For this review, take the finished solid that the model builds, in its own axes (mm). A direction names the side the tool comes from. Round coordinates to 2 decimals unless told otherwise and drop trailing zeros. Order: outer loops, then holes, each group sorted by start corner. A loop starts at its lowest first (then second) coordinate and runs counter-clockwise, first axis right, second up. Notation, with made-up numbers: M 81,65 L 123,65 A17 cw 123,95 Z; hole C 37.5,-8 d2. An arc over 180 degrees is marked long. Answer as a JSON object with one key per item and string values.
from build123d import *

# Parameters (mm, degrees)
BOSS_EXTRUDE1_DEPTH = 327.500000024


with BuildPart() as part:
    # Sketch1 → Boss-Extrude1 (new body)
    with BuildSketch(Plane.XY):
        Polygon((-22.499997904, -22.500007621), (-4.099997904, -22.500007621), (-4.099997904, -18.000007621), (-6.799997904, -18.000007621), (-6.799997904, -9.500007621), (-4.499997904, -7.200007621), (4.500002096, -7.200007621), (6.800002096, -9.500007621), (6.800002096, -18.000007621), (4.100002096, -18.000007621), (4.100002096, -22.500007621), (22.500002096, -22.500007621), (22.500002096, -4.100007621), (18.000002096, -4.100007621), (18.000002096, -6.800007621), (9.500002096, -6.800007621), (7.200002096, -4.500007621), (7.200002096, 4.499992379), (9.500002096, 6.799992379), (18.000002096, 6.799992379), (18.000002096, 4.099992379), (22.500002096, 4.099992379), (22.500002096, 22.499992379), (4.100002096, 22.499992379), (4.100002096, 17.999992379), (6.800002096, 17.999992379), (6.800002096, 9.499992379), (4.500002096, 7.199992379), (-4.499997904, 7.199992379), (-6.799997904, 9.499992379), (-6.799997904, 17.999992379), (-4.099997904, 17.999992379), (-4.099997904, 22.499992379), (-22.499997904, 22.499992379), (-22.499997904, 4.099992379), (-17.999997904, 4.099992379), (-17.999997904, 6.799992379), (-9.499997904, 6.799992379), (-7.199997904, 4.499992379), (-7.199997904, -4.500007621), (-9.499997904, -6.800007621), (-17.999997904, -6.800007621), (-17.999997904, -4.100007621), (-22.499997904, -4.100007621), align=None)
        Polygon((8.200003223, 8.199980186), (8.199989777, 19.399992368), (6.500002085, 19.399992368), (6.500002085, 21.099984758), (21.100004192, 21.099984758), (21.100004192, 6.499980188), (19.400009891, 6.499980188), (19.400009891, 8.199980186), align=None, mode=Mode.SUBTRACT)
        Polygon((-19.399997893, 6.499992368), (-21.099990283, 6.499992368), (-21.099990283, 21.099994475), (-6.499974376, 21.099994475), (-6.49997587, 19.399985233), (-8.199975868, 19.399986727), (-8.199985712, 8.19998006), (-19.399997893, 8.19998006), align=None, mode=Mode.SUBTRACT)
        Polygon((-6.499997893, -21.1), (-21.1, -21.1), (-21.1, -6.499995431), (-19.400002096, -6.499995431), (-19.400002096, -8.199995429), (-8.199995429, -8.199995429), (-8.199995429, -19.40000761), (-6.499997893, -19.400009104), align=None, mode=Mode.SUBTRACT)
        Polygon((6.499989905, -19.400011813), (8.199989903, -19.400011813), (8.199989903, -8.200005146), (19.400002085, -8.200005146), (19.400003579, -6.500017454), (21.099994475, -6.500018948), (21.099994475, -21.100009717), (6.499989905, -21.100009717), align=None, mode=Mode.SUBTRACT)
        with BuildLine():
            Line((-5.799999723, 3.537265469), (-3.451121085, 1.18838683))
            ThreePointArc((-3.451121085, 1.18838683), (-2.580942431, 2.580937072), (-1.188393996, 3.451118617))
            Line((-1.188393996, 3.451118617), (-3.537277512, 5.799992379))
            Line((-3.537277512, 5.799992379), (3.537277512, 5.799992379))
            Line((3.537277512, 5.799992379), (1.188393996, 3.451118617))
            ThreePointArc((1.188393996, 3.451118617), (2.580942431, 2.580937072), (3.451121085, 1.18838683))
            Line((3.451121085, 1.18838683), (5.799999723, 3.537265469))
            Line((5.799999723, 3.537265469), (5.799985034, -3.537266022))
            Line((5.799985034, -3.537266022), (3.451117181, -1.188398168))
            ThreePointArc((3.451117181, -1.188398168), (2.580938191, -2.580941312), (1.188393996, -3.451118617))
            Line((1.188393996, -3.451118617), (3.537277512, -5.799992379))
            Line((3.537277512, -5.799992379), (-3.537277512, -5.799992379))
            Line((-3.537277512, -5.799992379), (-1.188393996, -3.451118617))
            ThreePointArc((-1.188393996, -3.451118617), (-2.580938191, -2.580941311), (-3.451117181, -1.188398168))
            Line((-3.451117181, -1.188398168), (-5.799985034, -3.537266022))
            Line((-5.799985034, -3.537266022), (-5.799999723, 3.537265469))
        make_face(mode=Mode.SUBTRACT)
    extrude(amount=BOSS_EXTRUDE1_DEPTH)


solid = part.part
1) Insertion check: P1, Ø3, axis at y = 1, z = 275.5, coming from the +X side; P2, Ø3.5, axis at y = -1, z = 179.5, coming from the -X side. Each pin has a flat end and moves straight along its axis. Give the tip position at first contact, or say it passes through.
Geometry check:
{"P1": "stops at x = 7.2", "P2": "stops at x = -7.2"}
2) Machinability: for faces 1 (the flat face through (14, -6.8, 161)), 2 (the flat face through (22.5, 13, 161)), which of the approach directions +Z, -Z, +X, -X, +Y, -Y give a long, thin tool a straight path to every point of the face, cutting with its end or side? Answer none if there is none.
Geometry check:
{"face 1": "+Z, -Z", "face 2": "+Z, -Z, +X, +Y, -Y"}
3) Add section A-A on y = -14.5. State the section outline as (x, z) points, and give its area (3 significant figures).
Geometry check:
{"outline": "M -22.5,0 L -21.1,0 L -21.1,327.5 L -22.5,327.5 Z; M -8.2,0 L -6.8,0 L -6.8,327.5 L -8.2,327.5 Z; M 6.8,0 L 8.2,0 L 8.2,327.5 L 6.8,327.5 Z; M 21.1,0 L 22.5,0 L 22.5,327.5 L 21.1,327.5 Z", "area": "1,830 mm²"}
4) Mouldability with a two-part tool opening along Y and no side actions: class faces 3 (the flat face through (-14, -21.1, 161)), 4 (the flat face through (-13, -22.5, 161)), 5 (the flat face through (-3.4, 1.8, 327.5)) as +Y half, -Y half, draft (parallel to the pull), parting line (faces both ways), or undercut.
Geometry check:
{"face 3": "undercut", "face 4": "-Y half", "face 5": "draft"}
5) For L1, parallel to Y at x = 19, z = 20.5; L2, parallel to X at y = -17, z = 214; L3, parallel to X at y = 8.5, z = 112, list the stretches that pass through material, from the lowest coordinate up.
Geometry check:
{"L1": "y = -22.5 to -21.1, -8.2 to -4.1, 4.1 to 8.2, 21.1 to 22.5", "L2": "x = -22.5 to -21.1, -8.2 to -6.8, 6.8 to 8.2, 21.1 to 22.5", "L3": "x = -22.5 to -21.1, -8.2 to -5.8, 5.8 to 8.2, 21.1 to 22.5"}
6) Add section C-C on z = 65.5. State how many separate pieces and enclosed holes the cut face has, and give its area (3 significant figures).
Geometry check:
{"separate pieces": "1", "enclosed holes": "5", "area": "537 mm²"}
